The model under review builds one solid part; all positions refer to its coordinate system, in mm. A direction names the side the tool comes from. Give positions to 0.01 mm unless a question says otherwise; leave off trailing zeros. Order: outer loops, then holes, each group sorted by start corner. A loop starts at its lowest first (then second) coordinate and runs counter-clockwise, first axis right, second up. Notation, with made-up numbers: M -12.75,33 L -1.75,33 A26 cw -1.75,59 Z; hole C 89.5,73.25 d10. An arc over 180 degrees is marked long. One line per question, with ' | ' between items. Start each with the question number.
1. We need section C-C on z = -5.5. Write out the cut boundary in (x, y).
2. Insertion check: P1, Ø12, axis at x = -12.5, y = 17.5, coming from the -Z side; P2, Ø9, axis at x = -12, y = 16, coming from the +Z side; P3, Ø5, axis at x = 9, z = 4, coming from the +Y side. Each pin has a flat end and moves straight along its axis. Give the tip position at first contact, or say it passes through.
3. The part is to be moulded in two halves that separate along X. For faces 1 (the face through (19.844, 12, 0)), 2 (the face through (-1.45, 7.51, 1.89)), 3 (the face through (8, 12, 6.35)), say which applies: +X half, -X half, draft (parallel to the pull), parting line (faces both ways), or undercut.
4. Wall thickness on L1, parallel to Z at x = 0, y = 10.75: over which ranges is the line inside the solid? List them lowest first.
5. We need section B-B on x = 7. Write out the cut boundary in (y, z), then the cut area to 3 significant figures.
6. For faces 4 (the face through (-12, 14, -3.81)), 5 (the face through (11.988, 14.355, 3.219)), 6 (the face through (11.988, 8.823, -3.219)), list the 3-axis set-ups (+Z, -Z, +X, -X, +Y, -Y) from which the entire face can be reached by the end or side of a thin tool; tool diameter is ignored.
7. We need section D-D on y = 18. Write out the cut boundary in (x, z), then the cut area to 3 significant figures.
```python
from build123d import *

# Parameters (mm, degrees)
SKETCH1_R           = 6.35
BOSS_EXTRUDE1_DEPTH = 15.24
BOSS_EXTRUDE2_DEPTH = 19.84375
FILLET1_R           = 3.175
SKETCH3_R           = 2.38125
CUT_EXTRUDE1_DEPTH  = 26.813843458
BOSS_EXTRUDE3_DEPTH = 5.55625
BOSS_EXTRUDE4_DEPTH = 5.3975


with BuildPart() as part:
    # Sketch1 → Boss-Extrude1 (new body)
    with BuildSketch(Plane(origin=(0, 0, 0), x_dir=(1, 0, 0), z_dir=(0, 1, 0))):
        with Locations(Location((0, 0, 0), (0, 0, 90))):
            Circle(SKETCH1_R)
    extrude(amount=BOSS_EXTRUDE1_DEPTH)

    # Sketch2 → Boss-Extrude2 (add)
    with BuildSketch(Plane(origin=(0, 0, 0), x_dir=(0, 0, -1), z_dir=(1, 0, 0))):
        Polygon((-6.35, 9.68375), (-6.35, 13.49375), (0, 15.24), (6.35, 13.49375), (6.35, 9.68375), (0, 7.9375), align=None)
    extrude(amount=BOSS_EXTRUDE2_DEPTH)

    # Fillet1
    fillet1_edges = [part.edges().sort_by_distance(p)[0] for p in [
        (19.84375, 11.58875, 6.35),
        (19.84375, 11.58875, -6.35),
    ]]
    fillet(fillet1_edges, radius=FILLET1_R)

    # Sketch3 → Cut-Extrude1 (cut, through all)
    with BuildSketch(Plane.XZ):
        with Locations(Location((0, 0, 0), (0, 0, 270))):
            Circle(SKETCH3_R)
    extrude(amount=-CUT_EXTRUDE1_DEPTH, mode=Mode.SUBTRACT)

    # Sketch4 → Boss-Extrude3 (add)
    with BuildSketch(Plane(origin=(0, 15.24, 0), x_dir=(1, 0, 0), z_dir=(0, 1, 0))):
        with BuildLine():
            Line((-5.08, -3.81), (-16.03375, -3.81))
            ThreePointArc((-16.03375, -3.81), (-19.84375, 0), (-16.03375, 3.81))
            Line((-16.03375, 3.81), (-5.08, 3.81))
            ThreePointArc((-5.08, 3.81), (-6.35, 0), (-5.08, -3.81))
        make_face()
    extrude(amount=-BOSS_EXTRUDE3_DEPTH)

    # Sketch5 → Boss-Extrude4 (add)
    with BuildSketch(Plane(origin=(0, 15.24, 0), x_dir=(1, 0, 0), z_dir=(0, 1, 0))):
        with BuildLine():
            Line((-16.03375, 3.81), (-11.684, 3.81))
            ThreePointArc((-11.684, 3.81), (-7.874, 0), (-11.684, -3.81))
            Line((-11.684, -3.81), (-16.03375, -3.81))
            ThreePointArc((-16.03375, -3.81), (-19.84375, 0), (-16.03375, 3.81))
        make_face()
    extrude(amount=BOSS_EXTRUDE4_DEPTH)


solid = part.part
```
Entries:
1) outline: M -3.17,0 L 3.17,0 L 3.17,9.45 L 18.83,9.45 L 18.83,13.73 L 3.17,13.73 L 3.17,15.24 L -3.17,15.24 Z
2) P1: stops at z = -3.81 | P2: stops at z = 3.81 | P3: stops at y = 14.83
3) face 1: +X half | face 2: undercut | face 3: draft
4) L1: z = -6.35 to -2.38, 2.38 to 6.35
5) outline: M 7.94,0 L 9.68,-6.35 L 13.49,-6.35 L 15.24,0 L 13.49,6.35 L 9.68,6.35 Z | area: 70.6 mm^2
6) face 4: -Z, -X, +Y, -Y | face 5: +Z, +X, +Y | face 6: -Z, +X, -Y
7) outline: M -16.03,-3.81 L -11.68,-3.81 A3.81 ccw -11.68,3.81 L -16.03,3.81 A3.81 ccw Z | area: 78.7 mm^2
